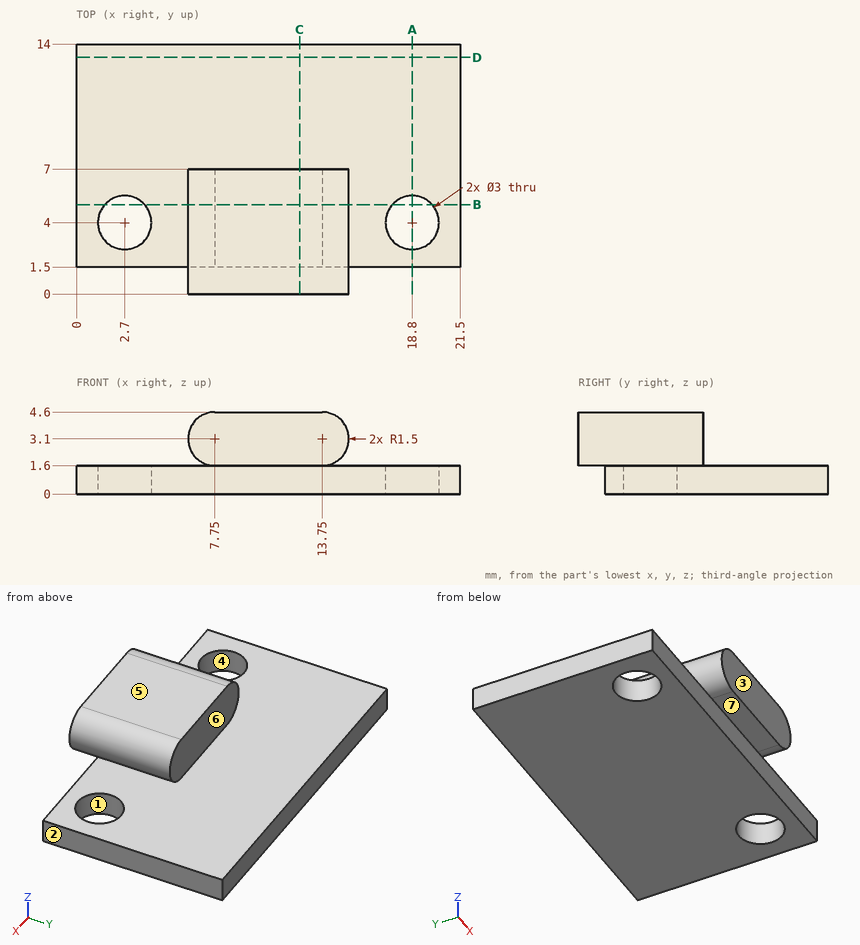
Input: dimensioned drawing with shaded views. Units: mm. Origin: part minimum x, y, z. A direction names the side the tool comes from. Coordinates: 2 decimals unless noted, no trailing zeros. Order: outer loops, then holes, each group sorted by start corner. A loop starts at its lowest first (then second) coordinate and runs counter-clockwise, first axis right, second up.
1. Cut plane C-C, the plane x = 12.5. Return loops of the section in (y, z), plus the area to 3 significant figures.
Checked values:
outline: (0, 1.6) - (1.5, 1.6) - (1.5, 0) - (14, 0) - (14, 1.6) - (7, 1.6) - (7, 4.6) - (0, 4.6) - close
area: 41.0 mm2
2. Contact query for flat-ended pins moving along their axis: P1, Ø1.5, axis at x = 10, z = 2.5, coming from the +Y side; P2, Ø0.8, axis at x = 6, z = 1, coming from the -Y side; P3, Ø6, axis at x = 19.5, y = 10.5, coming from the -Z side; P4, Ø4, axis at x = 2.7, y = 4, coming from the +Z side. Output: stop coordinate, or through.
Checked values:
P1: stops at y = 7
P2: stops at y = 1.5
P3: stops at z = 0
P4: stops at z = 1.6
3. Cut plane D-D, the plane y = 13.25. Return loops of the section in (x, z).
Checked values:
outline: (0, 0) - (21.5, 0) - (21.5, 1.6) - (0, 1.6) - close
4. Cut plane A-A, the plane x = 18.8. Return loops of the section in (y, z), plus the area to 3 significant figures.
Checked values:
outline: (1.5, 0) - (2.5, 0) - (2.5, 1.6) - (1.5, 1.6) - close; (5.5, 0) - (14, 0) - (14, 1.6) - (5.5, 1.6) - close
area: 15.2 mm2
5. Access query for the marked faces 5, 6 and 7. Directions: +Z, -Z, +X, -X, +Y, -Y. A direction counts if a zero-diameter tool reaches every point of the face in a straight line with its end or side. Return the directions, or none.
Checked values:
face 5: +Z, +X, -X, +Y, -Y
face 6: +Z, +X, -X, +Y
face 7: -Z, +X, -X, -Y
6. Cut plane B-B, the plane y = 5. Return loops of the section in (x, z), plus the area to 3 significant figures.
Checked values:
outline: (0, 0) - (1.58, 0) - (1.58, 1.6) - (0, 1.6) - close; (3.82, 0) - (17.68, 0) - (17.68, 1.6) - (13.75, 1.6) arc R1.5 ccw to (13.75, 4.6) - (7.75, 4.6) arc R1.5 ccw to (7.75, 1.6) - (3.82, 1.6) - close; (19.92, 0) - (21.5, 0) - (21.5, 1.6) - (19.92, 1.6) - close
area: 52.3 mm2
7. Ray query, line 1 along Y through (x, z) = (18.8, 0.7); line 2 along Z through (x, y) = (18.25, 7); line 3 along Y through (x, z) = (8.5, 1.5). Return the intervals inside material, ascending.
Checked values:
line 1: y = 1.5 to 2.5, 5.5 to 14
line 2: z = 0 to 1.6
line 3: y = 1.5 to 14
8. Draft query along Y for the marked faces 1, 2, 3 and 4. Return one class per face: +Y half, -Y half, draft (parallel to the pull), parting line (faces both ways), or undercut.
Checked values:
face 1: undercut
face 2: draft
face 3: -Y half
face 4: undercut
